Input: part model. Units: mm. Frame: model coordinates. A direction names the side the tool comes from. Coordinates: 2 decimals unless noted, no trailing zeros. Order: outer loops, then holes, each group sorted by start corner. A loop starts at its lowest first (then second) coordinate and runs counter-clockwise, first axis right, second up. Notation, with made-up numbers: (-20, 4) - (35, 4) arc R32 cw to (35, 34) - close; hole circle Ø9 at (44, 54.5). An arc over 180 degrees is marked (long way). Answer as CSV lines item,"result". Start each with the question number.
Item 1: Access query for faces 1 (the cylindrical face through (112.05, -38.59, 5.75)), 2 (the flat face through (110, -36, -2.377)), 3 (the cylindrical face through (18.845, -35.74, -30.001)), 4 (the flat face through (64, -36.5, 5)), 5 (the flat face through (110, -36, 14.112)). Directions: +Z, -Z, +X, -X, +Y, -Y. A direction counts if a zero-diameter tool reaches every point of the face in a straight line with its end or side. Return the directions, or none.
Item 2: Material intervals for line 1 along Y through (x, z) = (77, -0.5); line 2 along X through (y, z) = (-35.8, -8.5); line 3 along Z through (x, y) = (108, -35.35), sorted ascending.
Item 3: First-contact query: pin 1 (1.6 mm diameter, centred on y = -38, z = 6, fed in from -X); pin 2 (1.2 mm diameter, centred on y = -35.5, z = -16, fed in from +X); pin 3 (10 mm diameter, centred on x = 71, z = 10.5, fed in from -Y). Flat tips, straight axial feed; report the tip coordinate or a pass-through.
Item 4: Section C-C (x = 76). Output: boundary loops of the cut face in (y, z), and give its area (3 significant figures).
Item 5: Section B-B (z = 8). Output: boundary loops of the cut face in (x, y), and give its area (3 significant figures).
Item 6: Section A-A (y = -35.8). Output: boundary loops of the cut face in (x, z), and give its area (3 significant figures).
Item 7: Section D-D (z = -10). Output: boundary loops of the cut face in (x, y), and give its area (3 significant figures).
from build123d import *

# Parameters (mm, degrees)
BOSS_EXTRUDE1_DEPTH = 1.5
SKETCH3_W           = 16.488499631
SKETCH3_H           = 1.5
BOSS_EXTRUDE2_DEPTH = 8
SKETCH4_W           = 2.982324071
SKETCH4_H           = 16.488499631
REVOLVE1_ANGLE      = 90
FILLET1_R           = 1


with BuildPart() as part:
    # Sketch2 → Boss-Extrude1 (new body)
    with BuildSketch(Plane(origin=(0, -35, 0), x_dir=(1, 0, 0), z_dir=(0, 1, 0))):
        with BuildLine():
            Line((21.347125896, 31.053674712), (101.402209804, 31.053674712))
            ThreePointArc((101.402209804, 31.053674712), (103.877083539, 30.028548446), (104.902209804, 27.553674712))
            Line((104.902209804, 27.553674712), (104.902209804, -39.288548186))
            ThreePointArc((104.902209804, -39.288548186), (103.877083539, -41.76342192), (101.402209804, -42.788548186))
            Line((101.402209804, -42.788548186), (21.347125896, -42.788548186))
            ThreePointArc((21.347125896, -42.788548186), (18.872252162, -41.76342192), (17.847125896, -39.288548186))
            Line((17.847125896, -39.288548186), (17.847125896, 27.553674712))
            ThreePointArc((17.847125896, 27.553674712), (18.872252162, 30.028548446), (21.347125896, 31.053674712))
        make_face()
    extrude(amount=-BOSS_EXTRUDE1_DEPTH)

    # Sketch3 → Boss-Extrude2 (add)
    with BuildSketch(Plane(origin=(104.902209804, 0, 0), x_dir=(0, 0, -1), z_dir=(1, 0, 0))):
        with Locations((-5.867436738, -35.75)):
            Rectangle(SKETCH3_W, SKETCH3_H)
    extrude(amount=BOSS_EXTRUDE2_DEPTH)

    # Sketch4 → Revolve1 (revolve)
    with BuildSketch(Plane(origin=(0, -36.5, 0), x_dir=(-1, 0, 0), z_dir=(0, -1, 0))):
        with Locations((-111.411047768, -5.867436738)):
            Rectangle(SKETCH4_W, SKETCH4_H)
    revolve(axis=Axis((109.919885733, -36.5, 14.111686553), (0, 0, -1)), revolution_arc=REVOLVE1_ANGLE)

    # Fillet1
    fillet1_edges = [part.edges().sort_by_distance(p)[0] for p in [
        (109.919885733, -36.5, 5.867436737),
    ]]
    fillet(fillet1_edges, radius=FILLET1_R)


solid = part.part
Determined:
1,face 1,"+Z, -Z, +X, -Y"
1,face 2,"-Z, +X, +Y, -Y"
1,face 3,"-Z, -X, +Y, -Y"
1,face 4,"+Z, -Z, -X, -Y"
1,face 5,"+Z, +X, +Y, -Y"
2,line 1,"y = -36.5 to -35"
2,line 2,"x = 17.85 to 104.9"
2,line 3,"z = -2.38 to 14.11"
3,pin 1,"stops at x = 109.87"
3,pin 2,"stops at x = 104.9"
3,pin 3,"stops at y = -36.5"
4,outline,"(-36.5, -31.05) - (-35, -31.05) - (-35, 42.79) - (-36.5, 42.79) - close"
4,area,"111 mm^2"
5,outline,"(17.85, -36.5) - (108.92, -36.5) arc R1 cw to (109.92, -37.5) - (109.92, -39.48) arc R2.98 ccw to (112.9, -36.5) - (112.9, -35) - (17.85, -35) - close"
5,area,"150 mm^2"
6,outline,"(17.85, -27.55) arc R3.5 ccw to (21.35, -31.05) - (101.4, -31.05) arc R3.5 ccw to (104.9, -27.55) - (104.9, -2.38) - (112.9, -2.38) - (112.9, 14.11) - (104.9, 14.11) - (104.9, 39.29) arc R3.5 ccw to (101.4, 42.79) - (21.35, 42.79) arc R3.5 ccw to (17.85, 39.29) - close"
6,area,"6,550 mm^2"
7,outline,"(17.85, -36.5) - (104.9, -36.5) - (104.9, -35) - (17.85, -35) - close"
7,area,"131 mm^2"
